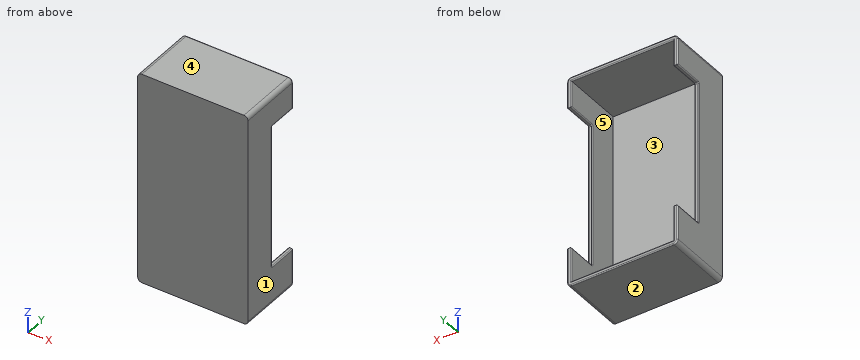
Autodesk Inventor part; units mm, degrees
ref_plane "YZ Plane" through (0, 0, 0) normal (1, 0, 0) x (0, 1, 0)
ref_plane "XZ Plane" through (0, 0, 0) normal (0, 1, 0) x (-1, 0, 0)
ref_plane "XY Plane" through (0, 0, 0) normal (0, 0, 1) x (1, 0, 0)
sketch "Sketch1" plane through (0, 0, 0) normal (0, 1, 0) x (-1, 0, 0)
  line L0 (50, 2) -> (0, 2)
  line L1 (-2, 0) -> (-2, -100)
  line L2 (0, -102) -> (50, -102)
  line L3 (52, -100) -> (52, 0)
  arc A0 (52, 0) -> (50, 2) centre (50, 0) ccw
  arc A1 (0, 2) -> (-2, 0) centre (0, 0) ccw
  arc A2 (-2, -100) -> (0, -102) centre (0, -100) ccw
  arc A3 (50, -102) -> (52, -100) centre (50, -100) ccw
  line L4 (50, 0) -> (0, 0)
  line L5 (0, 0) -> (0, -100)
  line L6 (0, -100) -> (50, -100)
  line L7 (50, -100) -> (50, 0)
  point P0 (0, 0)
  point P1 (50, -100)
  point P2 (50, 0)
  point P3 (0, -100)
  dimension "d0" = 50
  dimension "d1" = 100
  dimension "d7" = 2
  dimension "d8" = 100
  dimension "d9" = 2
  dimension "d10" = 2
  dimension "d11" = 2
  dimension "d12" = 2
  dimension "d13" = 50
extrude "Extrusion1" add sketch "Sketch1" along normal blind 2 contours A0 L3 A3 L2 A2 L1 A1 L0 | L7 L6 L5 L4
extrude "Extrusion2" add sketch "Sketch1" along normal blind 32
sketch "Sketch2" plane through (0, 32, 0) normal (0, 1, 0) x (1, 0, 0)
  arc A0 (0, -2) -> (2, 0) centre (0, 0) ccw
  line L0 (2, 0) -> (2, 100)
  arc A1 (2, 100) -> (0, 102) centre (0, 100) ccw
  line L1 (0, 102) -> (-50, 102)
  arc A2 (-50, 102) -> (-52, 100) centre (-50, 100) ccw
  line L2 (-52, 100) -> (-52, 0)
  arc A3 (-52, 0) -> (-50, -2) centre (-50, 0) ccw
  line L3 (-50, -2) -> (0, -2)
  line L4 (-50, 0) -> (-50, 100)
  line L5 (-50, 100) -> (0, 100)
  line L6 (0, 100) -> (0, 0)
  line L7 (0, 0) -> (-50, 0)
  line L8 (-50, 0) -> (0, 0)
  line L9 (0, 0) -> (0, 100)
  line L10 (0, 100) -> (-50, 100)
  line L11 (-50, 100) -> (-50, 0)
  line L12 (-52, 100) -> (-52, 0)
  line L13 (-52, 13) -> (-50, 13)
  line L14 (-50, 13) -> (-50, 83)
  line L15 (-50, 83) -> (-52, 83)
  line L16 (-52, 83) -> (-52, 13)
  line L17 (0, 13) -> (2, 13)
  line L18 (2, 13) -> (2, 83)
  line L19 (2, 83) -> (0, 83)
  line L20 (0, 83) -> (0, 13)
  point P0 (0, 0)
  point P1 (-52, 48)
  point P2 (0, 83)
  dimension "d18" = 2
  dimension "d19" = 70
  dimension "d20" = 50
extrude "Extrusion3" cut sketch "Sketch2" against normal blind 15 contours L17 L6 L19 L0 | L2 L15 L4 L13
fillet "Fillet1" radius 0.5 32 edges at (-52, 17, -48) (-50, 17, -48) (0, 17, -48) (2, 17, -48) (2, 24.5, -83) (0, 24.5, -83) (1, 17, -83) (1, 17, -13) (0, 24.5, -13) (2, 24.5, -13) (-50, 24.5, -83) (-52, 24.5, -83) (-51, 17, -83) (-50, 24.5, -13) (-52, 24.5, -13) (-51, 17, -13) (-50, 32, -91.5) (-51.4142, 32, -101.4142) (-25, 32, -102) (1.4142, 32, -101.4142) (2, 32, -91.5) (-52, 32, -91.5) (-25, 32, -100) (0, 32, -91.5) (1.4142, 32, 1.4142) (-25, 32, 2) (-51.4142, 32, 1.4142) (-52, 32, -6.5) (2, 32, -6.5) (0, 32, -6.5) (-25, 32, 0) (-50, 32, -6.5)
properties part number "connection box"
The listing builds one solid part. Answer for the finished solid, in the listing's coordinates (mm). Face numbers are marked on the shaded views. A direction names the side the tool comes from. Coordinates: 2 decimals unless noted, no trailing zeros. Loops run counter-clockwise (first coordinate to the right, second up) from the corner with the lowest first, then second, coordinate; pieces in that order, holes last. Notation, with made-up numbers: (37.25, 80) - (44.25, 80) arc R13 ccw to (44.25, 105) - close; hole circle Ø4 at (65, -30). An arc over 180 degrees is marked (long way). Use a Markdown table: item, result. Add a question column.
1) The part is cut by section B-B, the plane z = -54.5. Give the vertices of the cut face in (x, y).
2) For the marked faces 4 and 5, determine the directions among +Z, -Z, +X, -X, +Y, -Y from which every point of the face is accessible in a straight line to the end or side of a thin tool.
3) The part is cut by section C-C, the plane y = 26. Give the vertices of the cut face in (x, z), and give its area (3 significant figures).
4) Find the intervals of material crossed by line 1 (X direction, y = 7.5, z = -89.5); line 2 (Z direction, x = -32, y = 4); line 3 (Y direction, x = -24, z = -67.5), in increasing order.
5) The part is cut by section A-A, the plane y = 12.5. Give the vertices of the cut face in (x, z), and give its area (3 significant figures).
6) The part is cut by section D-D, the plane x = -1.5. Give the vertices of the cut face in (y, z), and give its area (3 significant figures).
7) Given pin 1 (1.1 mm diameter, centred on x = -51, z = -65, fed in from +Y); pin 2 (10 mm diameter, centred on x = -8, z = -58, fed in from +Y); pin 3 (0.8 mm diameter, centred on x = -51, y = 25, fed in from +Z), each flat-ended and moving along its own axis, determine where each tip first touches the part or whether it passes through.
8) The mould has two halves that part along Z. Classify the marked faces 1, 2 and 3: released by +Z, released by -Z, zero draft, split by the parting line, or undercut.
Here are the results:
| question | item | result |
|---|---|---|
| 1 | outline | (-52, 0) - (2, 0) - (2, 16.5) arc R0.5 ccw to (1.5, 17) - (0.5, 17) arc R0.5 ccw to (0, 16.5) - (0, 2) - (-50, 2) - (-50, 16.5) arc R0.5 ccw to (-50.5, 17) - (-51.5, 17) arc R0.5 ccw to (-52, 16.5) - close |
| 2 | face 4 | +Z, +X, -X, +Y, -Y |
| 2 | face 5 | +Y |
| 3 | outline | (-52, -100) arc R2 ccw to (-50, -102) - (0, -102) arc R2 ccw to (2, -100) - (2, -83.5) arc R0.5 ccw to (1.5, -83) - (0.5, -83) arc R0.5 ccw to (0, -83.5) - (0, -100) - (-50, -100) - (-50, -83.5) arc R0.5 ccw to (-50.5, -83) - (-51.5, -83) arc R0.5 ccw to (-52, -83.5) - close; (-52, -12.5) arc R0.5 ccw to (-51.5, -13) - (-50.5, -13) arc R0.5 ccw to (-50, -12.5) - (-50, 0) - (0, 0) - (0, -12.5) arc R0.5 ccw to (0.5, -13) - (1.5, -13) arc R0.5 ccw to (2, -12.5) - (2, 0) arc R2 ccw to (0, 2) - (-50, 2) arc R2 ccw to (-52, 0) - close |
| 3 | area | 332 mm^2 |
| 4 | line 1 | x = -52 to -50, 0 to 2 |
| 4 | line 2 | z = -102 to -100, 0 to 2 |
| 4 | line 3 | y = 0 to 2 |
| 5 | outline | (-52, -100) arc R2 ccw to (-50, -102) - (0, -102) arc R2 ccw to (2, -100) - (2, 0) arc R2 ccw to (0, 2) - (-50, 2) arc R2 ccw to (-52, 0) - close; hole (-50, -100) - (0, -100) - (0, 0) - (-50, 0) - close |
| 5 | area | 613 mm^2 |
| 6 | outline | (0, -102) - (31.5, -102) arc R0.5 ccw to (32, -101.5) - (32, -100.5) arc R0.5 ccw to (31.5, -100) - (2, -100) - (2, 0) - (31.5, 0) arc R0.5 ccw to (32, 0.5) - (32, 1.5) arc R0.5 ccw to (31.5, 2) - (0, 2) - close |
| 6 | area | 328 mm^2 |
| 7 | pin 1 | stops at y = 17 |
| 7 | pin 2 | stops at y = 2 |
| 7 | pin 3 | stops at z = 1.91 |
| 8 | face 1 | zero draft |
| 8 | face 2 | released by -Z |
| 8 | face 3 | undercut |
